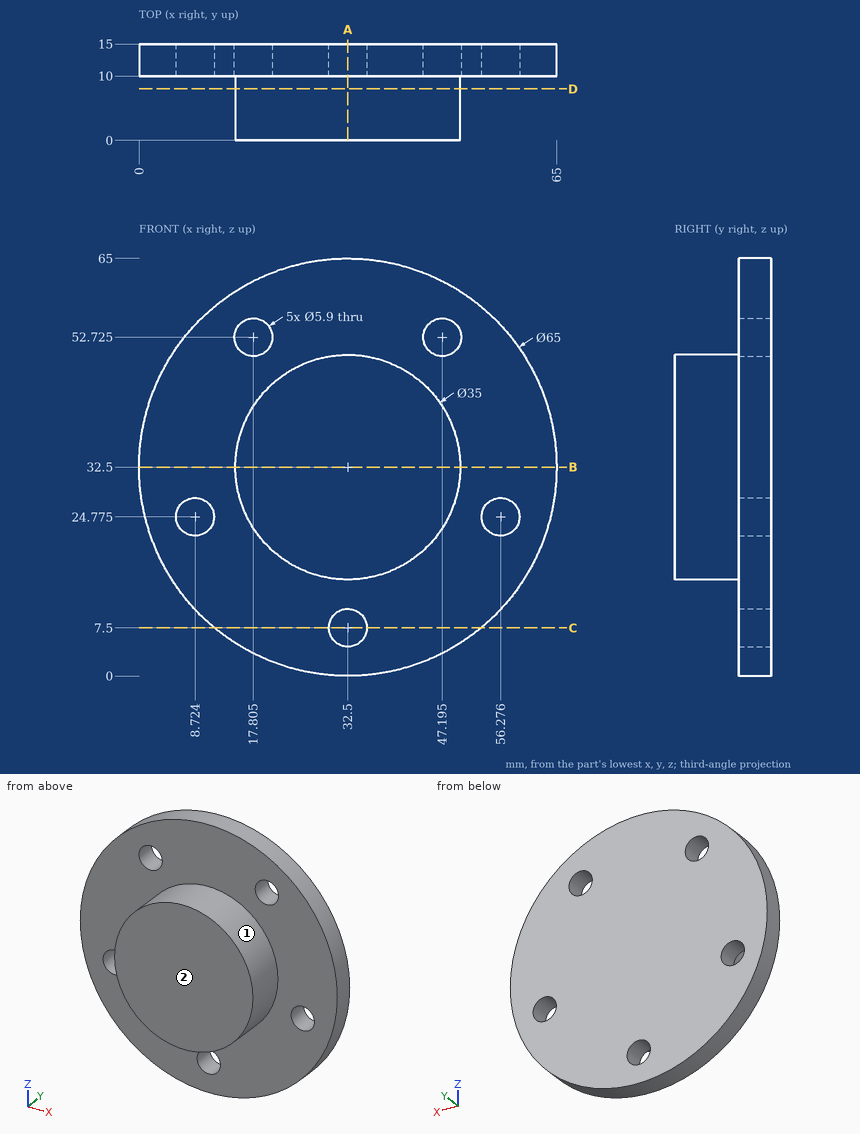
Input: dimensioned drawing with shaded views. Units: mm. Origin: part minimum x, y, z. A direction names the side the tool comes from. Give positions to 0.01 mm unless a question says otherwise; leave off trailing zeros. Write each loop counter-clockwise with the first axis right and the second up, starting at its lowest first coordinate (ties: lowest second). Pieces come first, ordered by that corner, then holes. Notation, with made-up numbers: M 19.25,33 L 70.25,33 A21 cw 70.25,68 Z; hole C -1.5,-38 d2. An arc over 180 degrees is marked long. Write item = value, one per line. Start each with the question number.
1) Material intervals for line 1 along Y through (x, z) = (3.5, 22.5); line 2 along Z through (x, y) = (33.5, 13.5) (1 decimal); line 3 along X through (y, z) = (10.25, 19.5), sorted ascending. Write a range as [from, to].
2) Cut plane B-B on z = 32.5. Return the cut outline in (x, y).
3) Cut plane A-A on x = 32.5. Return the cut outline in (y, z).
4) Reachability of the marked faces 1 and 2 from +Z, -Z, +X, -X, +Y, -Y: full face, straight path, thin tool, end or side. Return the list, or none.
5) Cut plane D-D on y = 8. Return the cut outline in (x, z).
6) First-contact query: pin 1 Ø3.5 at (x, z) = (47.19, 52.73) entering from -Y (1 decimal); pin 2 Ø2 at (y, z) = (7.5, 29.5) entering from +X (1 decimal); pin 3 Ø1 at (x, z) = (18, 14.5) entering from -Y. Flat tips, straight axial feed; report the tip coordinate or a pass-through.
7) Cut plane C-C on z = 7.5. Return the cut outline in (x, y), then the cut area to 3 significant figures.
Solved:
q1.line_1 = [10, 15]
q1.line_2 = [0, 4.7], [10.3, 65]
q1.line_3 = [2.71, 62.29]
q2.outline = M 0,10 L 15,10 L 15,0 L 50,0 L 50,10 L 65,10 L 65,15 L 0,15 Z
q3.outline = M 0,15 L 10,15 L 10,10.45 L 15,10.45 L 15,65 L 10,65 L 10,50 L 0,50 Z; M 10,0 L 15,0 L 15,4.55 L 10,4.55 Z
q4.face_1 = -Y
q4.face_2 = +Z, -Z, +X, -X, -Y
q5.outline = C 32.5,32.5 d35
q6.pin_1 = through
q6.pin_2 = 49.9
q6.pin_3 = 10
q7.outline = M 11.73,10 L 29.55,10 L 29.55,15 L 11.73,15 Z; M 35.45,10 L 53.27,10 L 53.27,15 L 35.45,15 Z
q7.area = 178 mm2
